```python
from build123d import *

# Parameters (mm, degrees)
F1_DEPTH = 8
F3_W     = 18.096443
F3_H     = 7.978035
F5_DEPTH = 8
F4_W     = 18.115349
F4_H     = 7.803778
F6_DEPTH = 8


with BuildPart() as f1:
    # F0 (on Top) → F1 (new body)
    with BuildSketch(Plane.XY):
        with BuildLine():
            ThreePointArc((54.546267, -5.591677), (57.887006, 0), (54.546267, 5.591677))
            Line((54.546267, 5.591677), (-27.175577, 49.571755))
            ThreePointArc((-27.175577, 49.571755), (-33.441654, 49.431285), (-36.534838, 43.980078))
            Line((-36.534838, 43.980078), (-36.534838, -43.980078))
            ThreePointArc((-36.534838, -43.980078), (-33.441654, -49.431285), (-27.175577, -49.571755))
            Line((-27.175577, -49.571755), (54.546267, -5.591677))
        make_face()
    extrude(amount=F1_DEPTH)

    # F3 (on face) → F5 (cut)
    with BuildSketch(Plane.XY.offset(8)):
        with Locations((-1.760172, 26.635416)):
            Rectangle(F3_W, F3_H)
    extrude(amount=-F5_DEPTH, mode=Mode.SUBTRACT)

    # F4 (on face) → F6 (cut)
    with BuildSketch(Plane.XY.offset(8)):
        with Locations((-1.75072, -26.947488)):
            Rectangle(F4_W, F4_H)
    extrude(amount=-F6_DEPTH, mode=Mode.SUBTRACT)


solid = f1.part
```
Could you check a few things on this model? Use its own coordinates, in mm. A direction names the side the tool comes from. Round coordinates to 2 decimals unless told otherwise and drop trailing zeros. Write each loop counter-clockwise with the first axis right and the second up, starting at its lowest first coordinate (ties: lowest second). Pieces come first, ordered by that corner, then holes. Notation, with made-up numbers: M -32.5,41 L 12.5,41 A7 ccw 12.5,46 Z; hole C 1,0.5 d9. An arc over 180 degrees is marked long. Write each question's results on one line, items separated by ' | '. Start each with the question number.
1. Imagine slicing it at C-C on y = -16. List the corners of the cut face in (x, z) for me, and give its area (3 significant figures).
2. I'm going to push flat-ended pins straight in: pin 1 Ø2 at (x, z) = (-26.5, 3) entering from +Y; pin 2 Ø2.5 at (x, z) = (-1.5, 4) entering from -Y; pin 3 Ø2.5 at (x, z) = (-3, 4.5) entering from +Y. Where does each tip first touch, or does it pass through?
3. I need wall thicknesses on L1, parallel to Y at x = 6, z = 4.5; L2, parallel to Y at x = 5.5, z = 4.5; L3, parallel to X at y = 23.5, z = 1.25. Which ranges of each line are inside material? Lowest first, please. Write a range as from..to.
4. Imagine slicing it at A-A on z = 2.5. List the corners of the cut face in (x, y) for me.
5. Imagine slicing it at D-D on x = -12.5. List the corners of the cut face in (y, z) for me.
6. Imagine slicing it at B-B on x = -2.5. List the corners of the cut face in (y, z) for me, and give its area (3 significant figures).
7. Thinking about a two-plate mould opening in Y: for faces 1 (the face through (-2, -30.849, 4)), 2 (the face through (-33.52, -49.384, 3.944)), 3 (the face through (14.257, 27.274, 3.944)), which applies, +Y half, -Y half, draft (parallel to the pull), parting line (faces both ways), or undercut?
8. On a 3-axis mill with a long thin cutter (end or side, diameter ignored), from which of +Z, -Z, +X, -X, +Y, -Y can I reach the whole of each face in a straight line? I mean faces 4 (the face through (-2, -23.046, 4)), 5 (the face through (57.886, -0.096, 3.944)). Say none if no direction works.
Result sheet:
1) outline: M -36.53,0 L 35.21,0 L 35.21,8 L -36.53,8 Z | area: 574 mm^2
2) pin 1: stops at y = 49.73 | pin 2: stops at y = -36.43 | pin 3: stops at y = 37.23
3) L1: y = -31.72..-30.85, -23.05..22.65, 30.62..31.72 | L2: y = -31.99..-30.85, -23.05..22.65, 30.62..31.99 | L3: x = -36.53..-10.81, 7.29..21.27
4) outline: M -36.53,-43.98 A6.35 ccw -27.18,-49.57 L 54.55,-5.59 A6.35 ccw 54.55,5.59 L -27.18,49.57 A6.35 ccw -36.53,43.98 Z; hole M -10.81,-30.85 L 7.31,-30.85 L 7.31,-23.05 L -10.81,-23.05 Z; hole M -10.81,22.65 L 7.29,22.65 L 7.29,30.62 L -10.81,30.62 Z
5) outline: M -41.67,0 L 41.67,0 L 41.67,8 L -41.67,8 Z
6) outline: M -36.29,0 L -30.85,0 L -30.85,8 L -36.29,8 Z; M -23.05,0 L 22.65,0 L 22.65,8 L -23.05,8 Z; M 30.62,0 L 36.29,0 L 36.29,8 L 30.62,8 Z | area: 454 mm^2
7) face 1: undercut | face 2: -Y half | face 3: +Y half
8) face 4: +Z, -Z | face 5: +Z, -Z, +X
